The listing builds one solid part. Answer for the finished solid, in the listing's coordinates (mm). A direction names the side the tool comes from. Give positions to 0.01 mm unless a question says otherwise; leave off trailing zeros. Write each loop counter-clockwise with the first axis right and the second up, starting at its lowest first coordinate (ties: lowest second). Pieces come first, ordered by that corner, then holes. Notation, with made-up numbers: (82, 3) - (92, 3) arc R13 ccw to (92, 18) - close; hole circle Ø2 at (12, 62.5). An arc over 180 degrees is marked (long way). Return JSON: item names as keys, results as strings.
from build123d import *

# Parameters (mm, degrees)
EXTRUDE_1_DEPTH      = 5
EXTRUDE_1_DEPTH_BACK = 5
FILLET_1_R           = 1
MM_CLEARANCE_1_D     = 2


with BuildPart() as part:
    # Sketch 2 → Extrude 1 (new body, two sides)
    with BuildSketch(Plane.XY) as extrude_1_sk:
        Polygon((15.044070129, 19), (30, 19), (30, 14), (24, 14), (24, 10.5), (21.629319922, 10.5), align=None)
    extrude(amount=EXTRUDE_1_DEPTH)
    extrude(extrude_1_sk.sketch, amount=-EXTRUDE_1_DEPTH_BACK)

    # Fillet 1
    fillet_1_edges = [part.edges().sort_by_distance(p)[0] for p in [
        (15.044070129, 19, 0),
        (24, 14, 0),
    ]]
    fillet(fillet_1_edges, radius=FILLET_1_R)

    # mm Clearance _1 (through all)
    with Locations(Plane(origin=(0, 14, 0), x_dir=(-1, 0, 0), z_dir=(0, -1, 0))):
        with Locations((-27.5, 2.499999967), (-27.5, -2.500000033)):
            Hole(MM_CLEARANCE_1_D / 2)


solid = part.part
Item 1: A cutting plane is placed at B-B on y = 18. Determine the outline of the cut face in (x, z).
Answer below:
{"outline": "(16.08, -5) - (30, -5) - (30, 5) - (16.08, 5) - close; hole circle Ø2 at (27.5, -2.5); hole circle Ø2 at (27.5, 2.5)"}
Item 2: A cutting plane is placed at C-C on x = 27.5. Determine the outline of the cut face in (y, z), then the cut area to 3 significant figures.
Answer below:
{"outline": "(14, -5) - (19, -5) - (19, -3.5) - (14, -3.5) - close; (14, -1.5) - (19, -1.5) - (19, 1.5) - (14, 1.5) - close; (14, 3.5) - (19, 3.5) - (19, 5) - (14, 5) - close", "area": "30.0 mm²"}
Item 3: The mould has two halves that part along X. Classify faces 1 (the face through (28.424, 16.535, 2.883)), 2 (the face through (24.285, 13.699, -0.07)), 3 (the face through (23, 19, 0)): +X half, -X half, draft (parallel to the pull), parting line (faces both ways), or undercut.
Answer below:
{"face 1": "undercut", "face 2": "+X half", "face 3": "draft"}
Item 4: Flat-ended cylindrical pins translate along their axes: P1, Ø2.5, axis at x = 27.5, z = 2.5, coming from the -Y side; P2, Ø6, axis at x = 19, z = -2, coming from the -Y side; P3, Ø1, axis at y = 17, z = 0.5, coming from the -X side; P4, Ø3, axis at y = 12, z = -2.5, coming from the +X side. Find the tip coordinate at first contact, or state that the pin passes through.
Answer below:
{"P1": "stops at y = 14", "P2": "stops at y = 10.5", "P3": "stops at x = 16.22", "P4": "stops at x = 24.13"}
Item 5: A cutting plane is placed at D-D on z = 3.75. Determine the outline of the cut face in (x, y), then the cut area to 3 significant figures.
Answer below:
{"outline": "(16.29, 17.39) - (21.63, 10.5) - (24, 10.5) - (24, 13) arc R1 cw to (25, 14) - (30, 14) - (30, 19) - (17.08, 19) arc R1 ccw to start", "area": "77.4 mm²"}
Item 6: For faces 4 (the face through (28, 14, 0)), 5 (the face through (23, 10.5, 0)), determine the directions among +Z, -Z, +X, -X, +Y, -Y from which every point of the face is accessible in a straight line to the end or side of a thin tool.
Answer below:
{"face 4": "+Z, -Z, +X, -Y", "face 5": "+Z, -Z, +X, -X, -Y"}
Item 7: Consider L1, parallel to Z at x = 27.5, y = 16.65; L2, parallel to Y at x = 28.75, z = -3; L3, parallel to X at y = 17.75, z = 2.25. Determine where each line is inside the solid, lowest interval first.
Answer below:
{"L1": "z = -5 to -3.5, -1.5 to 1.5, 3.5 to 5", "L2": "y = 14 to 19", "L3": "x = 16.12 to 26.53, 28.47 to 30"}
Item 8: A cutting plane is placed at A-A on z = 2.5. Determine the outline of the cut face in (x, y).
Answer below:
{"outline": "(16.29, 17.39) - (21.63, 10.5) - (24, 10.5) - (24, 13) arc R1 cw to (25, 14) - (26.5, 14) - (26.5, 19) - (17.08, 19) arc R1 ccw to start; (28.5, 14) - (30, 14) - (30, 19) - (28.5, 19) - close"}
